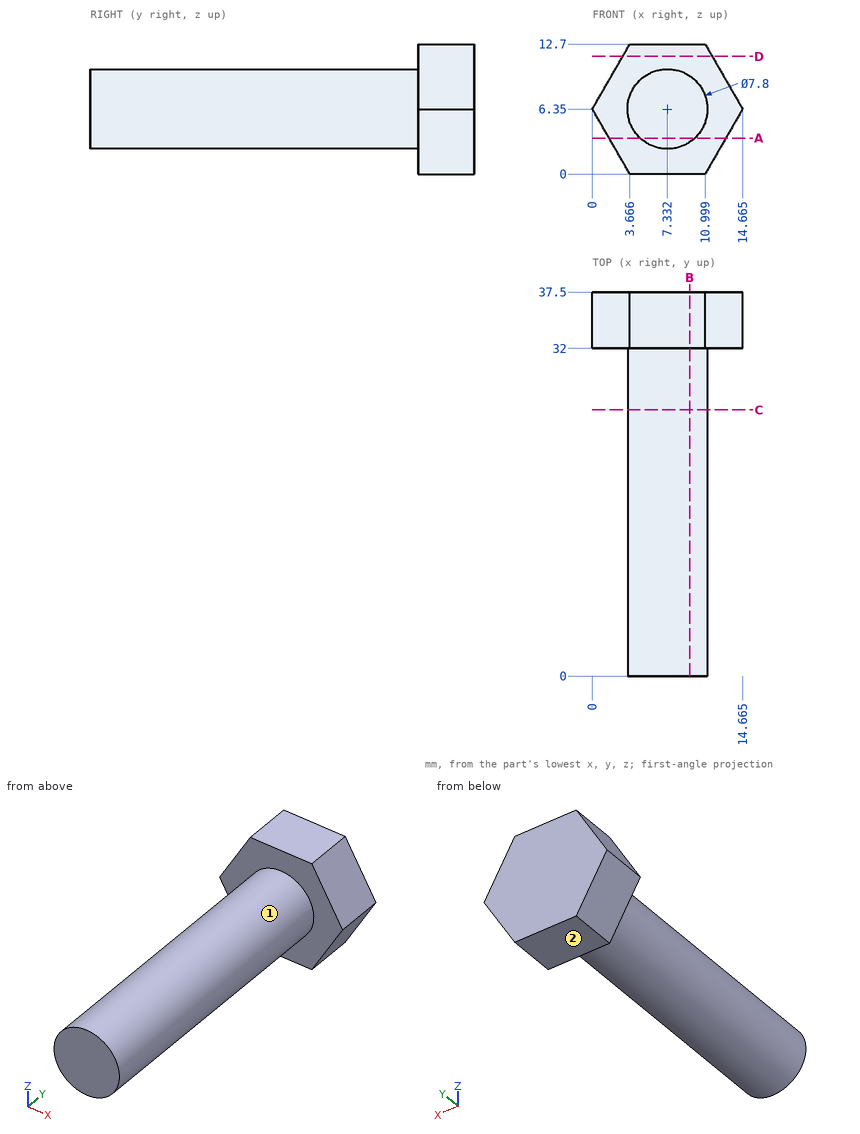
The figure shows three views and two pictorial views of one solid part (mm, origin at its lowest corner). Answer the questions. A direction names the side the tool comes from. Coordinates: 2 decimals unless noted, no trailing zeros. Loops run counter-clockwise (first coordinate to the right, second up) from the corner with the lowest first, then second, coordinate; pieces in that order, holes last. Notation, with made-up numbers: (30, -24.75) -> (55, -24.75) arc R27 ccw to (55, 4.25) -> close; hole circle Ø9 at (-35, -19). An arc over 180 degrees is marked (long way). Use one line per item in the form item = value. Start each with the question number.
Item 1: Consider L1, parallel to Y at x = 4.25, z = 1.5; L2, parallel to X at y = 21, z = 5 (1 decimal); L3, parallel to X at y = 17.5, z = 5.5 (1 decimal). Determine where each line is inside the solid, lowest interval first. Write a range as [from, to].
Item 2: The part is cut by section B-B on x = 9.5. Determine the outline of the cut face in (y, z).
Item 3: The part is cut by section A-A on z = 3.5. Determine the outline of the cut face in (x, y) (1 decimal).
Item 4: The part is cut by section C-C on y = 26. Determine the outline of the cut face in (x, z), then the cut area to 3 significant figures.
Item 5: A tool of negligible diameter and unlimited length cuts with its end or side. For the marked faces 1 and 2, from which of +Z, -Z, +X, -X, +Y, -Y can it reach the whole face along a straight path? Write none if from no direction.
Item 6: Flat-ended cylindrical pins translate along their axes: pin 1 Ø5 at (y, z) = (32.5, 9.5) entering from -X (1 decimal); pin 2 Ø2 at (x, y) = (9.5, 16) entering from -Z; pin 3 Ø2 at (x, y) = (4.5, 16) entering from -Z. Find the tip coordinate at first contact, or state that the pin passes through.
Item 7: The part is cut by section D-D on z = 11.5. Determine the outline of the cut face in (x, y).
Answer key:
q1.L1 = [32, 37.5]
q1.L2 = [3.7, 11]
q1.L3 = [3.5, 11.1]
q2.outline = (0, 3.11) -> (32, 3.11) -> (32, 0) -> (37.5, 0) -> (37.5, 12.7) -> (32, 12.7) -> (32, 9.59) -> (0, 9.59) -> close
q3.outline = (1.6, 32) -> (4.7, 32) -> (4.7, 0) -> (10, 0) -> (10, 32) -> (13, 32) -> (13, 37.5) -> (1.6, 37.5) -> close
q4.outline = circle Ø7.8 at (7.33, 6.35)
q4.area = 47.8 mm2
q5.face_1 = -Y
q5.face_2 = -Z, +X, -X, +Y, -Y
q6.pin_1 = 0.4
q6.pin_2 = 2.63
q6.pin_3 = 2.91
q7.outline = (2.97, 32) -> (11.69, 32) -> (11.69, 37.5) -> (2.97, 37.5) -> close
